Autodesk Inventor part; units mm, degrees
ref_plane "Work Plane1" through (0, 0, -3) normal (0, 0, -1) x (-1, 0, 0)
ref_plane "YZ Plane" through (0, 0, 0) normal (1, 0, 0) x (0, 1, 0)
ref_plane "XZ Plane" through (0, 0, 0) normal (0, 1, 0) x (-1, 0, 0)
ref_plane "Work Plane1" through (0, 0, -3) normal (0, 0, -1) x (-1, 0, 0)
sketch "Sketch1" plane through (0, 0, -3) normal (0, 0, -1) x (-1, 0, 0)
  line L0 (188.08, 47.916) -> (188.08, -47.916)
  line L1 (-110.3592, 171.5336) -> (188.08, 47.916)
  spline S0 degree 3 poles (-139.4832, 0) (-137.0244, 14.4817) (-134.5656, 28.9634) (-129.6218, 58.0812) (-127.1368, 72.7174) (-124.6518, 87.3535) (-122.1668, 101.99) (-119.6817, 116.6264) (-114.9175, 144.6864) (-112.6384, 158.11) (-110.3592, 171.5336) knots 0.047 0.047 0.047 0.047 4.453683 4.453683 8.907367 8.907367 8.907367 13.361137 13.361137 17.44584 17.44584 17.44584 17.44584
  spline S1 degree 3 poles (-110.3592, -171.5336) (-112.6384, -158.11) (-114.9175, -144.6864) (-119.6817, -116.6264) (-122.1668, -101.99) (-124.6518, -87.3535) (-127.1368, -72.7174) (-129.6218, -58.0812) (-134.5656, -28.9634) (-137.0244, -14.4817) (-139.4832, 0) knots 0.369067 0.369067 0.369067 0.369067 4.45377 4.45377 8.90754 8.90754 8.90754 13.361224 13.361224 17.767907 17.767907 17.767907 17.767907
  line L2 (188.08, -47.916) -> (-110.3592, -171.5336)
  point P0 (0, 0)
extrude "Extrusion1" add sketch "Sketch1" along normal blind 4
sketch "Sketch2" plane through (0, 0, -7) normal (0, 0, -1) x (-1, 0, 0)
  line L0 (188.08, -47.916) -> (188.08, 47.916) construction
  line L1 (188.08, 47.916) -> (-110.3592, 171.5336) construction
  line L2 (-110.3592, -171.5336) -> (188.08, -47.916) construction
  line L3 (138.08, 5) -> (188.08, 5)
  line L4 (188.08, 5) -> (188.08, -5)
  line L5 (188.08, -5) -> (138.08, -5)
  line L6 (138.08, -5) -> (138.08, 5)
  line L7 (99.2388, -30.5956) -> (90, -34.4224)
  line L8 (90, -34.4224) -> (109.1342, -80.6164)
  line L9 (109.1342, -80.6164) -> (118.373, -76.7896)
  line L10 (118.373, -76.7896) -> (99.2388, -30.5956)
  line L11 (-48.5819, -91.8249) -> (-57.8207, -95.6518)
  line L12 (-57.8207, -95.6518) -> (-38.6866, -141.8457)
  line L13 (-38.6866, -141.8457) -> (-29.4478, -138.0189)
  line L14 (-29.4478, -138.0189) -> (-48.5819, -91.8249)
  line L15 (-78.5805, -60) -> (-127.875, -68.3695)
  line L16 (-127.875, -68.3695) -> (-126.2011, -78.2284)
  line L17 (-126.2011, -78.2284) -> (-76.9066, -69.8589)
  line L18 (-76.9066, -69.8589) -> (-78.5805, -60)
  line L19 (-76.9066, 69.8589) -> (-126.2011, 78.2284)
  line L20 (-126.2011, 78.2284) -> (-127.875, 68.3695)
  line L21 (-127.875, 68.3695) -> (-78.5805, 60)
  line L22 (-78.5805, 60) -> (-76.9066, 69.8589)
  line L23 (109.1342, 80.6164) -> (118.373, 76.7896)
  line L24 (118.373, 76.7896) -> (99.2388, 30.5956)
  line L25 (99.2388, 30.5956) -> (90, 34.4224)
  line L26 (90, 34.4224) -> (109.1342, 80.6164)
  line L27 (188.08, -47.916) -> (188.08, 47.916)
  line L28 (-110.3592, -171.5336) -> (188.08, -47.916)
  line L29 (188.08, 47.916) -> (-110.3592, 171.5336)
  line L30 (-29.4478, 138.0189) -> (-38.6866, 141.8457)
  line L31 (-38.6866, 141.8457) -> (-57.8207, 95.6518)
  line L32 (-57.8207, 95.6518) -> (-48.5819, 91.8249)
  line L33 (-48.5819, 91.8249) -> (-29.4478, 138.0189)
  point P0 (0, 0)
  point P1 (-139.4832, 0)
  point P2 (188.08, 0)
  dimension "d2" = 10
  dimension "d3" = 10
  dimension "d5" = 10
  dimension "d6" = 10
  dimension "d7" = 10
  dimension "d8" = 10
  dimension "d10" = 50
  dimension "d11" = 50
  dimension "d12" = 50
  dimension "d13" = 50
  dimension "d14" = 50
  dimension "d15" = 50
  dimension "d18" = 150
  dimension "d19" = 60
  dimension "d20" = 60
  dimension "d21" = 90
  dimension "d22" = 90
  dimension "d23" = 10
  dimension "d24" = 50
  dimension "d25" = 150
extrude "Extrusion2" cut sketch "Sketch2" against normal through all
properties part number "internalSupportBottom2" material "Wood (Cherry)"
Source: CAD feature listing. Evaluate the final solid. Frame: model axes, mm. A direction names the side the tool comes from. Coordinates: 2 decimals unless noted, no trailing zeros. Order: outer loops, then holes, each group sorted by start corner. A loop starts at its lowest first (then second) coordinate and runs counter-clockwise, first axis right, second up. Notation, with made-up numbers: M -14,-39 L 13,-39 A29 cw 13,-1 Z; hole C 28.5,15.5 d2. An arc over 180 degrees is marked long. Write each question's results on one line, items separated by ' | '. Start each with the question number.
Item 1: Set-up query: faces 5 (the face through (14, 2, -3)), 6 (the face through (101.899, -74.102, -5.028)), 7 (the face through (39.15, 114.6, -5.03)). Return all of +Z, -Z, +X, -X, +Y, -Y with unobstructed straight access to the full face (end or side cutting, diameter ignored); none if empty.
Item 2: Draft query along X for faces 1 (the face through (103.573, 64.243, -5.028)), 2 (the face through (101.209, 73.985, -5.028)), 3 (the face through (48.12, 119.07, -5.03)), 4 (the face through (-38.87, 109.72, -4.97)). Return one class per face: pulls with the +X half, pulls with the -X half, needs draft (parallel to the pull), parting line crosses it, or undercut.
Item 3: Cut plane A-A (x = -127.5). Return loops of the section in (y, z), and give its area (3 significant figures).
Item 4: Cut plane B-B (x = -33). Return loops of the section in (y, z), and give its area (3 significant figures).
Item 5: Line query: probe 1 along Y at (x, z) = (50.5, -5.25); probe 2 along Y at (x, z) = (82, -5.75); probe 3 along Y at (x, z) = (-82, -4.25). Output: solid intervals per line, ascending.
Item 6: First-contact query: pin 1 Ø1.2 at (x, z) = (-157, -5.5) entering from -Y; pin 2 Ø1.5 at (x, z) = (33.5, -5.5) entering from +Y; pin 3 Ø2 at (x, z) = (-129.5, -4.5) entering from -Y. Flat tips, straight axial feed; report the tip coordinate or a pass-through.
Checked values:
1) face 5: +Z, +X, -X, +Y, -Y | face 6: +Z, -Z, +X | face 7: +Z, -Z
2) face 1: undercut | face 2: pulls with the +X half | face 3: undercut | face 4: pulls with the -X half
3) outline: M -73.01,-7 L 73.01,-7 L 73.01,-3 L -73.01,-3 Z | area: 584 mm2
4) outline: M -112.15,-7 L 112.15,-7 L 112.15,-3 L -112.15,-3 Z | area: 897 mm2
5) probe 1: y = -146.74 to -113.33, -92.62 to 92.62, 113.33 to 146.74 | probe 2: y = -159.79 to -70.72, -60.58 to 60.58, 70.72 to 159.79 | probe 3: y = -91.86 to 91.86
6) pin 1: stops at y = -61.04 | pin 2: stops at y = 130.05 | pin 3: stops at y = -72.59
